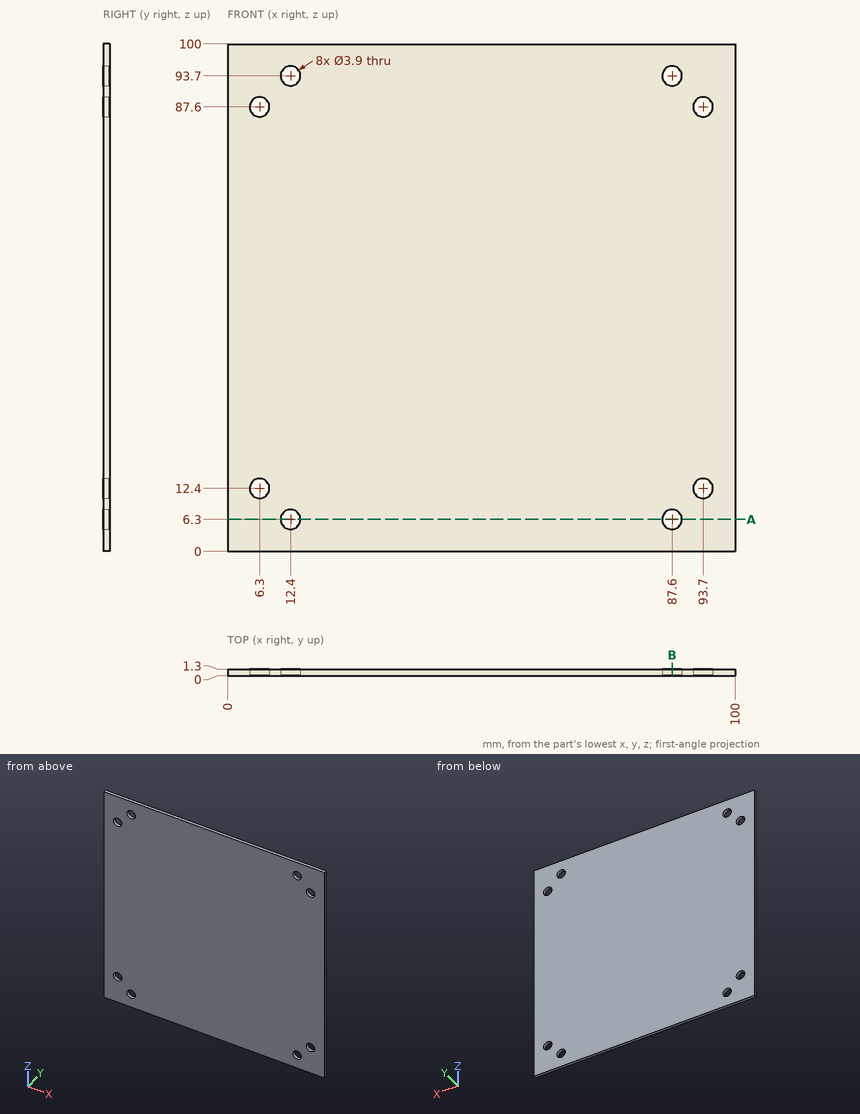
For this review, use the dimensioned drawing (mm, ordinates from the lowest corner) and the shaded views. Give positions to 0.01 mm unless a question says otherwise; leave off trailing zeros. Order: outer loops, then holes, each group sorted by start corner. A loop starts at its lowest first (then second) coordinate and runs counter-clockwise, first axis right, second up. Notation, with made-up numbers: (65, 85) - (120, 85) arc R29 cw to (120, 112) - close; hole circle Ø5 at (44.25, 60). An arc over 180 degrees is marked (long way). Use a Markdown table: item, result. Add a question column.
(1) Clearance check with a flat-ended pin moving along its axis: P1, Ø1.5, axis at x = 23.5, z = 50, coming from the -Y side. State where the tip first meets the part, or that it passes through.
(2) Wall thickness on probe 1 along X at (y, z) = (0.45, 6.3); probe 2 along X at (y, z) = (1.05, 12.4): over which ranges is each line inside the solid? List them lowest first. Write a range as [from, to].
(3) Add section B-B on x = 87.6. Give the boundary of the cut face in (y, z).
(4) Add section A-A on z = 6.3. Give the boundary of the cut face in (x, y), then the cut area to 3 significant figures.
Report:
| question | item | result |
|---|---|---|
| 1 | P1 | stops at y = 0 |
| 2 | probe 1 | x = [0, 10.45], [14.35, 85.65], [89.55, 100] |
| 2 | probe 2 | x = [0, 4.35], [8.25, 91.75], [95.65, 100] |
| 3 | outline | (0, 0) - (1.3, 0) - (1.3, 4.35) - (0, 4.35) - close; (0, 8.25) - (1.3, 8.25) - (1.3, 91.75) - (0, 91.75) - close; (0, 95.65) - (1.3, 95.65) - (1.3, 100) - (0, 100) - close |
| 4 | outline | (0, 0) - (10.45, 0) - (10.45, 1.3) - (0, 1.3) - close; (14.35, 0) - (85.65, 0) - (85.65, 1.3) - (14.35, 1.3) - close; (89.55, 0) - (100, 0) - (100, 1.3) - (89.55, 1.3) - close |
| 4 | area | 120 mm² |
